```python
from build123d import *

# Parameters (mm, degrees)
SKETCH2_R           = 0.24
BOSS_EXTRUDE1_DEPTH = 13


with BuildPart() as part:
    # Sketch1 → Revolve1 (revolve)
    with BuildSketch(Plane(origin=(0, 0, 0), x_dir=(1, 0, 0), z_dir=(0, 1, 0))):
        Polygon((0, 0), (4.6, 0), (4.6, 1), (4.13, 1), (4.13, 4.1), (3.63, 4.1), (3.63, 3.9), (0, 3.9), align=None)
    revolve(axis=Axis((0, 0, -3.9), (0, 0, 1)))

    # Sketch2 → Boss-Extrude1 (add)
    with BuildSketch(Plane.XY):
        with Locations((-2.54, 0)):
            Circle(SKETCH2_R)
        with Locations((2.54, 0)):
            Circle(SKETCH2_R)
    extrude(amount=BOSS_EXTRUDE1_DEPTH)


solid = part.part
```
The model under review builds one solid part; all positions refer to its coordinate system, in mm. Coordinates: 2 decimals unless noted, no trailing zeros. Order: outer loops, then holes, each group sorted by start corner. A loop starts at its lowest first (then second) coordinate and runs counter-clockwise, first axis right, second up. Notation, with made-up numbers: M 87.25,-28 L 146.25,-28 A3 ccw 146.25,-24 Z; hole C -15.5,72 d1. An arc over 180 degrees is marked long. One line per question, with ' | ' between items.
(1) The part is to be moulded in two halves that separate along Y. For faces 1 (the face through (0, 0, -3.9)), 2 (the face through (-3.65, -2.8, -0.51)), 3 (the face through (0, 0, 0)), say which applies: +Y half, -Y half, draft (parallel to the pull), parting line (faces both ways), or undercut.
Geometry results:
face 1: undercut | face 2: parting line | face 3: draft
(2) Insertion check: pin 1 (1 mm diameter, centred on x = -2.5, z = 1, fed in from +Y); pin 2 (4.5 mm diameter, centred on x = -1, y = 0, fed in from +Z); pin 3 (2 mm diameter, centred on y = -2, z = -2.5, fed in from -X); pin 4 (3 mm diameter, centred on y = 0, z = 2, fed in from +X). Each pin has a flat end and moves straight along its axis. Give the tip position at first contact, or say it passes through.
Geometry results:
pin 1: stops at y = 0.24 | pin 2: stops at z = 13 | pin 3: stops at x = -4.01 | pin 4: stops at x = 2.78
(3) Add section A-A, the plane y = 0. Write out the cut boundary in (x, z), then the cut area to 3 significant figures.
Geometry results:
outline: M -4.6,-1 L -4.13,-1 L -4.13,-4.1 L -3.63,-4.1 L -3.63,-3.9 L 3.63,-3.9 L 3.63,-4.1 L 4.13,-4.1 L 4.13,-1 L 4.6,-1 L 4.6,0 L 2.78,0 L 2.78,13 L 2.3,13 L 2.3,0 L -2.3,0 L -2.3,13 L -2.78,13 L -2.78,0 L -4.6,0 Z | area: 45.8 mm²
(4) Add section C-C, the plane z = 2.5. Write out the cut boundary in (x, y), then the cut area to 3 significant figures.
Geometry results:
outline: C -2.54,0 d0.48; C 2.54,0 d0.48 | area: 0.362 mm²
(5) Add section D-D, the plane x = 1.75. Write out the cut boundary in (y, z).
Geometry results:
outline: M -4.25,-1 L -3.74,-1 L -3.74,-4.1 L -3.18,-4.1 L -3.18,-3.9 L 3.18,-3.9 L 3.18,-4.1 L 3.74,-4.1 L 3.74,-1 L 4.25,-1 L 4.25,0 L -4.25,0 Z
(6) For probe 1 along Y at (x, z) = (0, -3.95); probe 2 along Z at (x, y) = (1.5, 0.75); probe 3 along Z at (x, y) = (3.75, 2.5), list the stretches that pass through material, from the lowest coordinate up. Write a range as from..to.
Geometry results:
probe 1: y = -4.13..-3.63, 3.63..4.13 | probe 2: z = -3.9..0 | probe 3: z = -1..0
(7) Add section B-B, the plane z = -1.5. Write out the cut boundary in (x, y).
Geometry results:
outline: C 0,0 d8.26
